Design review of the part built by this model. Coordinates are the model's own, in mm. Face numbers are marked on the shaded views. A direction names the side the tool comes from. Coordinates: 2 decimals unless noted, no trailing zeros. Loops run counter-clockwise (first coordinate to the right, second up) from the corner with the lowest first, then second, coordinate; pieces in that order, holes last. Notation, with made-up numbers: M -4,62.25 L 46,62.25 A26 ccw 46,101.25 Z; hole C -1,85 d5. An arc over 180 degrees is marked long. One line per item, written item: value.
```python
from build123d import *

# Parameters (mm, degrees)
SKETCH2_W           = 75
SKETCH2_H           = 8
SKETCH2_R           = 1.6
BOSS_EXTRUDE1_DEPTH = 2
SKETCH3_W           = 25
SKETCH3_H           = 18.5
BOSS_EXTRUDE2_DEPTH = 2
SKETCH4_W           = 25
SKETCH4_H           = 2
BOSS_EXTRUDE3_DEPTH = 18.5
SKETCH5_W           = 10.2
SKETCH5_H           = 40.2
CUT_EXTRUDE1_DEPTH  = 18.5
SKETCH6_W           = 10.2
SKETCH6_H           = 40.2
BOSS_EXTRUDE4_DEPTH = 24.9
SKETCH8_W           = 25
SKETCH8_H           = 7
BOSS_EXTRUDE5_DEPTH = 2
SKETCH9_R           = 1.6
CUT_EXTRUDE2_DEPTH  = 2
SKETCH10_W          = 20.2
SKETCH10_H          = 40.2
CUT_EXTRUDE3_DEPTH  = 77
SKETCH11_W          = 7
SKETCH11_H          = 2.4
CUT_EXTRUDE4_DEPTH  = 77
SKETCH12_W          = 2.4
SKETCH12_H          = 7
BOSS_EXTRUDE6_DEPTH = 24.9
SKETCH13_W          = 4
SKETCH13_H          = 4
CUT_EXTRUDE5_DEPTH  = 77
SKETCH14_W          = 25
SKETCH14_H          = 8
SKETCH14_R          = 1.6
BOSS_EXTRUDE7_DEPTH = 2
CUT_EXTRUDE6_DEPTH  = 2
CHAMFER1_SIZE       = 10
CUT_EXTRUDE7_DEPTH  = 1.2
SKETCH17_W          = 20.2
SKETCH17_H          = 22.9
CUT_EXTRUDE8_DEPTH  = 1.2
CUT_EXTRUDE9_DEPTH  = 2
CUT_EXTRUDE10_DEPTH = 2


with BuildPart() as part:
    # Sketch2 → Boss-Extrude1 (new body)
    with BuildSketch(Plane(origin=(0, 0, 0), x_dir=(1, 0, 0), z_dir=(0, 1, 0))):
        Rectangle(SKETCH2_W, SKETCH2_H)
        with Locations((-31.75, 0)):
            Circle(SKETCH2_R, mode=Mode.SUBTRACT)
        with Locations((31.75, 0)):
            Circle(SKETCH2_R, mode=Mode.SUBTRACT)
    extrude(amount=BOSS_EXTRUDE1_DEPTH)

    # Sketch3 → Boss-Extrude2 (add)
    with BuildSketch(Plane(origin=(0, 2, 0), x_dir=(1, 0, 0), z_dir=(0, 1, 0))):
        with Locations((0, -13.25)):
            Rectangle(SKETCH3_W, SKETCH3_H)
    extrude(amount=-BOSS_EXTRUDE2_DEPTH)

    # Sketch4 → Boss-Extrude3 (add)
    with BuildSketch(Plane(origin=(0, 0, -4), x_dir=(-1, 0, 0), z_dir=(0, 0, -1))):
        with Locations((0, 1)):
            Rectangle(SKETCH4_W, SKETCH4_H)
    extrude(amount=BOSS_EXTRUDE3_DEPTH)

    # Sketch5 → Cut-Extrude1 (cut)
    with BuildSketch(Plane(origin=(0, 2, 0), x_dir=(1, 0, 0), z_dir=(0, 1, 0))):
        Rectangle(SKETCH5_W, SKETCH5_H)
    extrude(amount=-CUT_EXTRUDE1_DEPTH, mode=Mode.SUBTRACT)

    # Sketch6 → Boss-Extrude4 (add)
    with BuildSketch(Plane(origin=(0, 2, 0), x_dir=(1, 0, 0), z_dir=(0, 1, 0))):
        Polygon((-12.5, 4), (-12.5, -4), (-12.5, -22.5), (12.5, -22.5), (12.5, -4), (12.5, 4), (12.5, 22.5), (-12.5, 22.5), align=None)
        Rectangle(SKETCH6_W, SKETCH6_H, mode=Mode.SUBTRACT)
    extrude(amount=BOSS_EXTRUDE4_DEPTH)

    # Sketch8 → Boss-Extrude5 (add)
    with BuildSketch(Plane(origin=(0, 26.9, 0), x_dir=(1, 0, 0), z_dir=(0, 1, 0))):
        with Locations((0, 26)):
            Rectangle(SKETCH8_W, SKETCH8_H)
        with Locations((0, -26)):
            Rectangle(SKETCH8_W, SKETCH8_H)
    extrude(amount=-BOSS_EXTRUDE5_DEPTH)

    # Sketch9 → Cut-Extrude2 (cut)
    with BuildSketch(Plane.XZ.offset(-24.9)):
        with Locations((5.2, 23.8)):
            Circle(SKETCH9_R)
        with Locations((-5.2, 23.8)):
            Circle(SKETCH9_R)
        with Locations((-5.2, -23.8)):
            Circle(SKETCH9_R)
        with Locations((5.2, -23.8)):
            Circle(SKETCH9_R)
    extrude(amount=-CUT_EXTRUDE2_DEPTH, mode=Mode.SUBTRACT)

    # Sketch10 → Cut-Extrude3 (cut)
    with BuildSketch(Plane.XZ):
        Rectangle(SKETCH10_W, SKETCH10_H)
    extrude(amount=-CUT_EXTRUDE3_DEPTH, mode=Mode.SUBTRACT)

    # Sketch11 → Cut-Extrude4 (cut)
    with BuildSketch(Plane.XZ):
        with Locations((0, -21.3)):
            Rectangle(SKETCH11_W, SKETCH11_H)
    extrude(amount=-CUT_EXTRUDE4_DEPTH, mode=Mode.SUBTRACT)

    # Sketch12 → Boss-Extrude6 (add)
    with BuildSketch(Plane.XZ):
        with Locations((-11.3, 26)):
            Rectangle(SKETCH12_W, SKETCH12_H)
        with Locations((-11.3, -26)):
            Rectangle(SKETCH12_W, SKETCH12_H)
        with Locations((11.3, 26)):
            Rectangle(SKETCH12_W, SKETCH12_H)
        with Locations((11.3, -26)):
            Rectangle(SKETCH12_W, SKETCH12_H)
    extrude(amount=-BOSS_EXTRUDE6_DEPTH)

    # Sketch13 → Cut-Extrude5 (cut)
    with BuildSketch(Plane(origin=(0, 26.9, 0), x_dir=(1, 0, 0), z_dir=(0, 1, 0))):
        with Locations((0, 22.5)):
            Rectangle(SKETCH13_W, SKETCH13_H)
    extrude(amount=-CUT_EXTRUDE5_DEPTH, mode=Mode.SUBTRACT)

    # Sketch14 → Boss-Extrude7 (add)
    with BuildSketch(Plane(origin=(0, 2, 0), x_dir=(1, 0, 0), z_dir=(0, 1, 0))):
        with Locations((-25, 0)):
            Rectangle(SKETCH14_W, SKETCH14_H)
        with Locations((-31.75, 0)):
            Circle(SKETCH14_R, mode=Mode.SUBTRACT)
        with Locations((25, 0)):
            Rectangle(SKETCH14_W, SKETCH14_H)
        with Locations((31.75, 0)):
            Circle(SKETCH14_R, mode=Mode.SUBTRACT)
    extrude(amount=BOSS_EXTRUDE7_DEPTH)

    # Sketch15 → Cut-Extrude6 (cut)
    with BuildSketch(Plane.XZ):
        Polygon((10.1, -20.1), (3.5, -20.1), (3.5, -22.5), (10.1, -22.5), (10.1, -29.5), (12.5, -29.5), (12.5, -4), (37.5, -4), (37.5, 4), (12.5, 4), (12.5, 29.5), (10.1, 29.5), (10.1, 22.5), (-10.1, 22.5), (-10.1, 29.5), (-12.5, 29.5), (-12.5, 4), (-37.5, 4), (-37.5, -4), (-12.5, -4), (-12.5, -29.5), (-10.1, -29.5), (-10.1, -22.5), (-3.5, -22.5), (-3.5, -20.1), (-10.1, -20.1), (-10.1, 20.1), (10.1, 20.1), align=None)
    extrude(amount=-CUT_EXTRUDE6_DEPTH, mode=Mode.SUBTRACT)

    # Chamfer1
    chamfer1_edges = [part.edges().sort_by_distance(p)[0] for p in [
        (-12.5, 4, 0),
        (12.5, 4, 0),
    ]]
    chamfer(chamfer1_edges, length=CHAMFER1_SIZE)

    # Sketch16 → Cut-Extrude7 (cut)
    with BuildSketch(Plane.XY.offset(22.5)):
        Polygon((-10.1, 2), (10.1, 2), (10.1, 24.9), (6.132737905, 24.9), (4.267262095, 24.9), (-4.267262095, 24.9), (-6.132737905, 24.9), (-10.1, 24.9), align=None)
    extrude(amount=-CUT_EXTRUDE7_DEPTH, mode=Mode.SUBTRACT)

    # Sketch17 → Cut-Extrude8 (cut)
    with BuildSketch(Plane(origin=(0, 0, -22.5), x_dir=(-1, 0, 0), z_dir=(0, 0, -1))):
        with Locations((0, 13.45)):
            Rectangle(SKETCH17_W, SKETCH17_H)
    extrude(amount=-CUT_EXTRUDE8_DEPTH, mode=Mode.SUBTRACT)

    # Sketch18 → Cut-Extrude9 (cut)
    with BuildSketch(Plane(origin=(0, 0, -29.5), x_dir=(-1, 0, 0), z_dir=(0, 0, -1))):
        Polygon((10.1, 2), (12.5, 2), (12.5, 26.9), (-12.5, 26.9), (-12.5, 2), (-10.1, 2), (-10.1, 24.9), (10.1, 24.9), align=None)
    extrude(amount=-CUT_EXTRUDE9_DEPTH, mode=Mode.SUBTRACT)

    # Sketch19 → Cut-Extrude10 (cut)
    with BuildSketch(Plane.XY.offset(29.5)):
        Polygon((10.1, 2), (12.5, 2), (12.5, 26.9), (-12.5, 26.9), (-12.5, 2), (-10.1, 2), (-10.1, 24.9), (10.1, 24.9), align=None)
    extrude(amount=-CUT_EXTRUDE10_DEPTH, mode=Mode.SUBTRACT)


solid = part.part
```
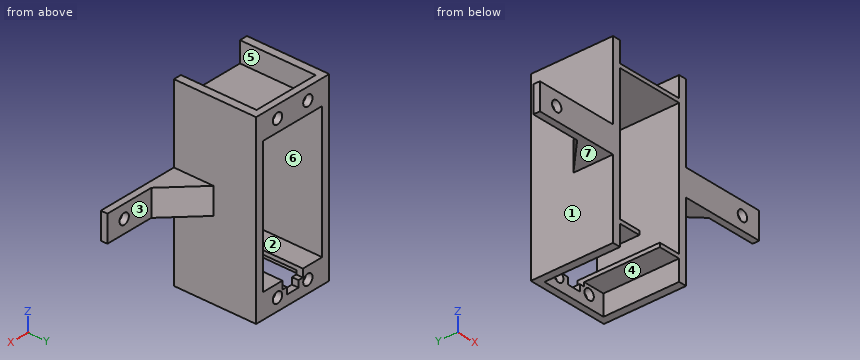
(1) Insertion check: pin 1 (12 mm diameter, centred on x = -29, z = -6.5, fed in from -Y); pin 2 (3 mm diameter, centred on x = -31.75, z = 0, fed in from +Y); pin 3 (4 mm diameter, centred on x = 27, z = -2, fed in from +Y); pin 4 (1.9 mm diameter, centred on y = 17.5, z = -25.5, fed in from +X). Each pin has a flat end and moves straight along its axis. Give the tip position at first contact, or say it passes through.
Reply:
pin 1: stops at y = 2
pin 2: passes through
pin 3: stops at y = 4
pin 4: stops at x = 12.5
(2) We need section C-C on x = -31.75. State the section outline as (y, z) points.
Reply:
outline: M 2,-4 L 4,-4 L 4,-1.6 L 2,-1.6 Z; M 2,1.6 L 4,1.6 L 4,4 L 2,4 Z
(3) To check wall thickness, follow line 1 along X through (y, z) = (3.15, 0); line 2 along Z through (x, y) = (-5.2, 25.5); line 3 along X through (y, z) = (21.5, -13.5). State the ranges of each line that lie inside material, in increasing order. Write a range as [from, to].
Reply:
line 1: x = [-37.5, -33.35], [-30.15, -10.1], [10.1, 30.15], [33.35, 37.5]
line 2: z = [-27.5, -25.4], [-22.2, -20.1], [20.1, 22.2], [25.4, 27.5]
line 3: x = [-12.5, -10.1], [10.1, 12.5]
(4) We need section D-D on y = 15.5. State the section outline as (x, z) points.
Reply:
outline: M -12.5,-27.5 L -10.1,-27.5 L -10.1,-21.3 L -3.5,-21.3 L -3.5,-20.1 L -10.1,-20.1 L -10.1,20.1 L 10.1,20.1 L 10.1,-20.1 L 3.5,-20.1 L 3.5,-21.3 L 10.1,-21.3 L 10.1,-27.5 L 12.5,-27.5 L 12.5,27.5 L 10.1,27.5 L 10.1,21.3 L -10.1,21.3 L -10.1,27.5 L -12.5,27.5 Z
(5) We need section B-B on z = 2.5. State the section outline as (x, y) points.
Reply:
outline: M -37.5,2 L -10.1,2 L -10.1,26.9 L -12.5,26.9 L -12.5,14 L -22.5,4 L -37.5,4 Z; M 10.1,2 L 37.5,2 L 37.5,4 L 22.5,4 L 12.5,14 L 12.5,26.9 L 10.1,26.9 Z
(6) Tool access review of the marked faces 4, 5, 6 and 7: name each direction out of +Z, -Z, +X, -X, +Y, -Y from which nothing blocks a thin tool from reaching the whole face with its end or side.
Reply:
face 4: -Z, -Y
face 5: +Z, -Y
face 6: +Y, -Y
face 7: -Z, -X, +Y, -Y
(7) Mouldability with a two-part tool opening along X and no side actions: class the marked faces 1, 2 and 3 as released by +X, released by -X, zero draft, split by the parting line, or undercut.
Reply:
face 1: released by -X
face 2: undercut
face 3: zero draft
(8) We need section A-A on x = -5.2. State the section outline as (y, z) points, then the cut area to 3 significant figures.
Reply:
outline: M 2,-21.3 L 24.9,-21.3 L 24.9,-22.2 L 26.9,-22.2 L 26.9,-20.1 L 2,-20.1 Z; M 2,20.1 L 26.9,20.1 L 26.9,22.2 L 24.9,22.2 L 24.9,21.3 L 2,21.3 Z; M 24.9,-27.5 L 26.9,-27.5 L 26.9,-25.4 L 24.9,-25.4 Z; M 24.9,25.4 L 26.9,25.4 L 26.9,27.5 L 24.9,27.5 Z
area: 71.8 mm2
